For this review, take the finished solid that the model builds, in its own axes (mm). Round coordinates to 2 decimals unless told otherwise and drop trailing zeros. Order: outer loops, then holes, each group sorted by start corner. A loop starts at its lowest first (then second) coordinate and runs counter-clockwise, first axis right, second up. Notation, with made-up numbers: M 61.25,42 L 80.25,42 A21 cw 80.25,70 Z; hole C 76,27.5 d2. An arc over 180 degrees is marked long. Answer as a JSON object with one key per item and string values.
Autodesk Inventor part; units mm, degrees
ref_plane "YZ Plane" through (0, 0, 0) normal (1, 0, 0) x (0, 1, 0)
ref_plane "XZ Plane" through (0, 0, 0) normal (0, 1, 0) x (-1, 0, 0)
ref_plane "XY Plane" through (0, 0, 0) normal (0, 0, 1) x (1, 0, 0)
sketch "Sketch1" plane through (0, 0, 0) normal (0, 0, 1) x (1, 0, 0)
  line L0 (-88.9, -57.15) -> (88.9, -57.15)
  line L1 (88.9, -57.15) -> (88.9, 57.15)
  line L2 (88.9, 57.15) -> (-88.9, 57.15)
  line L3 (-88.9, 57.15) -> (-88.9, -57.15)
  line L4 (-40, -6.35) -> (40, -6.35)
  line L5 (40, -6.35) -> (40, 6.35)
  line L6 (40, 6.35) -> (-40, 6.35)
  line L7 (-40, 6.35) -> (-40, -6.35)
  point P0 (-35, 0)
  point P1 (-20, 0)
  dimension "d0" = 177.8
  dimension "d1" = 114.3
  dimension "d2" = 80
  dimension "d3" = 12.7
extrude "Extrusion1" add sketch "Sketch1" along normal blind 12.7 contours L3 L2 L1 L0 | L7 L6 L5 L4
hole "Hole1" at (-35, 0, 0) at (-20, 0, 0) direction (0, 0, 1) diameter 5 end through all
properties part number "LoadCellLowerSide"
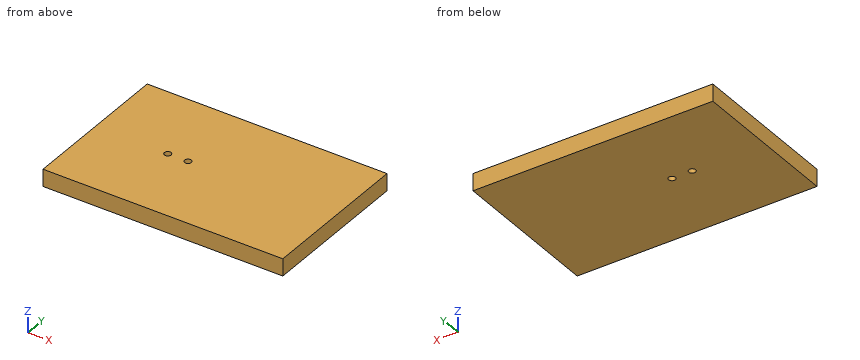
1) For L1, parallel to X at y = 0, z = 6.75; L2, parallel to Y at x = -20, z = 6.25; L3, parallel to Y at x = -20.5, z = 11.75, list the stretches that pass through material, from the lowest coordinate up.
Geometry check:
{"L1": "x = -88.9 to -37.5, -32.5 to -22.5, -17.5 to 88.9", "L2": "y = -57.15 to -2.5, 2.5 to 57.15", "L3": "y = -57.15 to -2.45, 2.45 to 57.15"}
2) Add section A-A on x = -20. State the section outline as (y, z) points, and give its area (3 significant figures).
Geometry check:
{"outline": "M -57.15,0 L -2.5,0 L -2.5,12.7 L -57.15,12.7 Z; M 2.5,0 L 57.15,0 L 57.15,12.7 L 2.5,12.7 Z", "area": "1,390 mm²"}
3) Add section B-B on y = 0. State the section outline as (x, z) points, and give its area (3 significant figures).
Geometry check:
{"outline": "M -88.9,0 L -37.5,0 L -37.5,12.7 L -88.9,12.7 Z; M -32.5,0 L -22.5,0 L -22.5,12.7 L -32.5,12.7 Z; M -17.5,0 L 88.9,0 L 88.9,12.7 L -17.5,12.7 Z", "area": "2,130 mm²"}
4) Insertion check: P1, Ø6.5, axis at x = -35, y = 0, coming from the +Z side. The pin has a flat end and moves straight along its axis. Give the tip position at first contact, or say it passes through.
Geometry check:
{"P1": "stops at z = 12.7"}
